The listing builds one solid part. Answer for the finished solid, in the listing's coordinates (mm). Face numbers are marked on the shaded views. A direction names the side the tool comes from. Give positions to 0.01 mm unless a question says otherwise; leave off trailing zeros. Write each loop counter-clockwise with the first axis right and the second up, starting at its lowest first coordinate (ties: lowest second). Pieces come first, ordered by that corner, then holes. Notation, with made-up numbers: (-35, 83.25) - (-9, 83.25) arc R14 ccw to (-9, 106.25) - close; hole circle Ø2 at (43, 82). An arc over 180 degrees is marked (long way). Return JSON: item names as keys, results as strings.
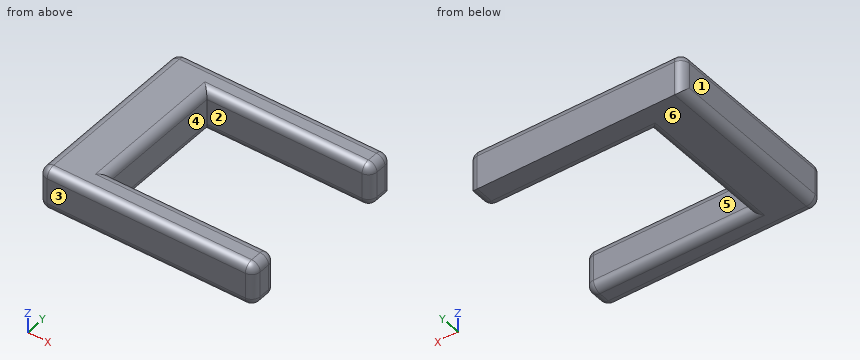
from build123d import *

# Parameters (mm, degrees)
F0_W     = 30.1708392799
F0_H     = 76.7637714744
F1_DEPTH = 25.4
F2_R     = 5.08


with BuildPart() as f1:
    # F0 (on Top) → F1 (new body)
    with BuildSketch(Plane.XY):
        with Locations((-48.0250958353, -0.8592940867)):
            Rectangle(F0_W, F0_H)
        Polygon((-32.9396761954, -39.2411798239), (-63.1105154753, -39.2411798239), (-63.1105154753, -56.0451894999), (65.4019713402, -56.0451894999), (65.4019713402, -39.2411798239), align=None)
        Polygon((64.8291036487, 53.9446882904), (-63.1105154753, 53.9446882904), (-63.1105154753, 37.5225916505), (-32.9396761954, 37.5225916505), (64.8291036487, 37.5225916505), align=None)
    extrude(amount=F1_DEPTH)

    # F2
    f2_edges = [f1.edges().sort_by_distance(p)[0] for p in [
        (15.944714, 37.522592, 25.4),
        (-32.939676, -0.859294, 25.4),
        (16.231148, -39.24118, 25.4),
        (65.401971, -47.643185, 25.4),
        (64.829104, 45.73364, 25.4),
        (1.145728, -56.045189, 25.4),
        (65.401971, -56.045189, 12.7),
        (65.401971, -39.24118, 12.7),
        (-63.110515, -56.045189, 12.7),
        (-63.110515, -1.050251, 25.4),
        (0.859294, 53.944688, 25.4),
        (64.829104, 37.522592, 12.7),
        (64.829104, 53.944688, 12.7),
        (-63.110515, 53.944688, 12.7),
        (-63.110515, -1.050251, 0),
        (1.145728, -56.045189, 0),
        (15.944714, 37.522592, 0),
        (-32.939676, -0.859294, 0),
        (16.231148, -39.24118, 0),
        (65.401971, -47.643185, 0),
        (64.829104, 45.73364, 0),
    ]]
    fillet(f2_edges, radius=F2_R)


solid = f1.part
Item 1: For the marked faces 1 and 2, determine the directions among +Z, -Z, +X, -X, +Y, -Y from which every point of the face is accessible in a straight line to the end or side of a thin tool.
Answer below:
{"face 1": "+Z, -Z, -X, +Y, -Y", "face 2": "+Z, -Z, +X"}
Item 2: A cutting plane is placed at C-C on z = 14.75. Determine the outline of the cut face in (x, y), then the cut area to 3 significant figures.
Answer below:
{"outline": "(-63.11, -50.97) arc R5.08 ccw to (-58.03, -56.05) - (60.32, -56.05) arc R5.08 ccw to (65.4, -50.97) - (65.4, -44.32) arc R5.08 ccw to (60.32, -39.24) - (-32.94, -39.24) - (-32.94, 37.52) - (59.75, 37.52) arc R5.08 ccw to (64.83, 42.6) - (64.83, 48.86) arc R5.08 ccw to (59.75, 53.94) - (-58.03, 53.94) arc R5.08 ccw to (-63.11, 48.86) - close", "area": "6,540 mm²"}
Item 3: Consider L1, parallel to Y at x = -31, z = 18.75; L2, parallel to X at y = -42, z = 9; L3, parallel to Y at x = 50, z = 3.5. Determine where each line is inside the solid, lowest interval first.
Answer below:
{"L1": "y = -56.05 to -39.24, 37.52 to 53.94", "L2": "x = -63.11 to 64.84", "L3": "y = -55.79 to -39.49, 37.77 to 53.94"}
Item 4: The mould has two halves that part along Y. Classify the marked faces 3, 4, 5 and 6: +Y half, -Y half, draft (parallel to the pull), parting line (faces both ways), or undercut.
Answer below:
{"face 3": "-Y half", "face 4": "undercut", "face 5": "undercut", "face 6": "draft"}
Item 5: A cutting plane is placed at D-D on z = 3.25. Determine the outline of the cut face in (x, y).
Answer below:
{"outline": "(-62.77, -50.97) arc R4.74 ccw to (-58.03, -55.7) - (60.32, -55.7) arc R4.74 ccw to (65.06, -50.97) - (65.06, -44.32) arc R4.74 ccw to (60.32, -39.58) - (-33.28, -39.58) - (-33.28, 37.86) - (59.75, 37.86) arc R4.74 ccw to (64.49, 42.6) - (64.49, 50.69) arc R5.08 ccw to (59.75, 53.94) - (-58.03, 53.94) arc R5.08 ccw to (-62.77, 50.69) - close"}
Item 6: Flat-ended cylindrical pins translate along their axes: P1, Ø7, axis at y = 44, z = 9, coming from the +X side; P2, Ø4, axis at x = -24, z = 22.5, coming from the +Y side; P3, Ø8, axis at y = 11, z = 15.5, coming from the +X side. Find the tip coordinate at first contact, or state that the pin passes through.
Answer below:
{"P1": "stops at x = 64.83", "P2": "stops at y = 53.94", "P3": "stops at x = -32.94"}
Item 7: A cutting plane is placed at A-A on x = -31. Determine the outline of the cut face in (y, z).
Answer below:
{"outline": "(-56.05, 5.08) arc R5.08 ccw to (-50.97, 0) - (-44.32, 0) arc R5.08 ccw to (-39.24, 5.08) - (-39.24, 20.32) arc R5.08 ccw to (-44.32, 25.4) - (-50.97, 25.4) arc R5.08 ccw to (-56.05, 20.32) - close; (37.52, 5.08) arc R5.08 ccw to (42.6, 0) - (53.94, 0) - (53.94, 20.32) arc R5.08 ccw to (48.86, 25.4) - (42.6, 25.4) arc R5.08 ccw to (37.52, 20.32) - close"}
Item 8: A cutting plane is placed at B-B on y = 25. Determine the outline of the cut face in (x, z), then the cut area to 3 significant figures.
Answer below:
{"outline": "(-63.11, 5.08) arc R5.08 ccw to (-58.03, 0) - (-38.02, 0) arc R5.08 ccw to (-32.94, 5.08) - (-32.94, 20.32) arc R5.08 ccw to (-38.02, 25.4) - (-58.03, 25.4) arc R5.08 ccw to (-63.11, 20.32) - close", "area": "744 mm²"}
